Check sheet for the modelled part. Datum: model origin and axes. Units: mm. Round coordinates to 2 decimals unless told otherwise and drop trailing zeros. Order: outer loops, then holes, each group sorted by start corner. A loop starts at its lowest first (then second) coordinate and runs counter-clockwise, first axis right, second up.
```python
from build123d import *

# Parameters (mm, degrees)
F1_DEPTH     = 300
F2_R         = 15
F4_DEPTH     = 1
F5_T1_DEPTH  = 260
F5_T3_DEPTH  = 114.4173096389
F5_T5_DEPTH  = 114.4173096389
F5_T8_ANGLE  = 90
F5_T10_ANGLE = 90
F5_T12_ANGLE = 90
F5_T14_ANGLE = 90
F7_DEPTH     = 0.1
F9_DEPTH     = 0.1


# Not quite as in the source:
# - a fillet or chamfer that OpenCascade refuses, or shapes differently, is made with other operations: its cross-section is extruded or revolved along the edge and cut away or added


with BuildPart() as f1:
    # F0 (on Right) → F1 (new body)
    with BuildSketch(Plane.YZ):
        Polygon((-104.210527479, 1), (-104.210527479, 0), (115.789472521, 0), (115.789472521, 10), align=None)
    extrude(amount=F1_DEPTH)

    # F2
    f2_edges = [f1.edges().sort_by_distance(p)[0] for p in [
        (300, 115.789473, 5),
        (0, 115.789473, 5),
        (0, -104.210527, 0.5),
        (300, -104.210527, 0.5),
    ]]
    fillet(f2_edges, radius=F2_R)

    # F3 (on face) → F4 (cut)
    with BuildSketch(Plane(origin=(0, -0.2149512742, 5.2543644811), x_dir=(1, 0, 0), z_dir=(0, -0.040874902, 0.999164272))):
        with BuildLine():
            Line((280, 101.0889066279), (20, 101.0889066279))
            ThreePointArc((20, 101.0889066279), (16.4644660941, 99.6244405339), (15, 96.0889066279))
            Line((15, 96.0889066279), (15, -18.328403011))
            ThreePointArc((15, -18.328403011), (16.4644660941, -21.8639369169), (20, -23.328403011))
            Line((20, -23.328403011), (280, -23.328403011))
            ThreePointArc((280, -23.328403011), (283.5355339059, -21.8639369169), (285, -18.328403011))
            Line((285, -18.328403011), (285, 96.0889066279))
            ThreePointArc((285, 96.0889066279), (283.5355339059, 99.6244405339), (280, 101.0889066279))
        make_face()
    extrude(amount=-F4_DEPTH, mode=Mode.SUBTRACT)

    # F5: fillet of radius 5 on 8 edges, made by hand

    # F5_s2 → F5_t1 (join)
    with BuildSketch(Plane.YZ.offset(20)):
        with BuildLine():
            ThreePointArc((100.789472521, 9.3863636364), (99.4021842094, 8.5855726288), (97.8328546072, 8.2645746583))
            Line((97.8328546072, 8.2645746583), (100.8303474231, 8.3871993644))
            Line((100.8303474231, 8.3871993644), (100.789472521, 9.3863636364))
        make_face()
        with BuildLine():
            ThreePointArc((-23.5238580849, 4.3008182934), (-22.0757956208, 3.6160189085), (-20.485490367, 3.4242787275))
            Line((-20.485490367, 3.4242787275), (-23.4829831829, 3.3016540214))
            Line((-23.4829831829, 3.3016540214), (-23.5238580849, 4.3008182934))
        make_face()
    extrude(amount=F5_T1_DEPTH)

    # F5_s4 → F5_t3 (join)
    with BuildSketch(Plane(origin=(0, 96.0086024354, 3.9276246451), x_dir=(1, 0, 0), z_dir=(0, -0.999164272, -0.040874902))):
        with BuildLine():
            ThreePointArc((15, 5.2587593737), (16.4188611699, 4.5153428835), (18, 4.2587593737))
            Line((18, 4.2587593737), (15, 4.2587593737))
            Line((15, 4.2587593737), (15, 5.2587593737))
        make_face()
    extrude(amount=F5_T3_DEPTH)

    # F5_s6 → F5_t5 (join)
    with BuildSketch(Plane(origin=(0, -18.3130854508, -0.7491716775), x_dir=(1, 0, 0), z_dir=(0, 0.999164272, 0.040874902))):
        with BuildLine():
            ThreePointArc((285, -5.2587593737), (283.5811388301, -4.5153428835), (282, -4.2587593737))
            Line((282, -4.2587593737), (285, -4.2587593737))
            Line((285, -4.2587593737), (285, -5.2587593737))
        make_face()
    extrude(amount=F5_T5_DEPTH)

    # F5_s7 → F5_t8 (revolve)
    with BuildSketch(Plane.YZ.offset(20)):
        with BuildLine():
            ThreePointArc((100.789472521, 9.3863636364), (99.4021842094, 8.5855726288), (97.8328546072, 8.2645746583))
            Line((97.8328546072, 8.2645746583), (100.8303474231, 8.3871993644))
            Line((100.8303474231, 8.3871993644), (100.789472521, 9.3863636364))
        make_face()
    revolve(axis=Axis((20, 95.8345260632, 8.1828248542), (0, -0.040874902, 0.999164272)), revolution_arc=F5_T8_ANGLE)

    # F5_s9 → F5_t10 (revolve)
    with BuildSketch(Plane(origin=(0, -18.3130854508, -0.7491716775), x_dir=(1, 0, 0), z_dir=(0, 0.999164272, 0.040874902))):
        with BuildLine():
            ThreePointArc((15, -5.2587593737), (16.4188611699, -4.5153428835), (18, -4.2587593737))
            Line((18, -4.2587593737), (15, -4.2587593737))
            Line((15, -4.2587593737), (15, -5.2587593737))
        make_face()
    revolve(axis=Axis((20, -18.487161823, 3.5060285316), (0, -0.040874902, 0.999164272)), revolution_arc=F5_T10_ANGLE)

    # F5_s11 → F5_t12 (revolve)
    with BuildSketch(Plane.YZ.offset(280)):
        with BuildLine():
            ThreePointArc((-23.5238580849, 4.3008182934), (-22.0757956208, 3.6160189085), (-20.485490367, 3.4242787275))
            Line((-20.485490367, 3.4242787275), (-23.4829831829, 3.3016540214))
            Line((-23.4829831829, 3.3016540214), (-23.5238580849, 4.3008182934))
        make_face()
    revolve(axis=Axis((280, -18.487161823, 3.5060285316), (0, -0.040874902, 0.999164272)), revolution_arc=F5_T12_ANGLE)

    # F5_s13 → F5_t14 (revolve)
    with BuildSketch(Plane(origin=(0, 96.0086024354, 3.9276246451), x_dir=(1, 0, 0), z_dir=(0, -0.999164272, -0.040874902))):
        with BuildLine():
            ThreePointArc((285, 5.2587593737), (283.5811388301, 4.5153428835), (282, 4.2587593737))
            Line((282, 4.2587593737), (285, 4.2587593737))
            Line((285, 4.2587593737), (285, 5.2587593737))
        make_face()
    revolve(axis=Axis((280, 95.8345260632, 8.1828248542), (0, -0.040874902, 0.999164272)), revolution_arc=F5_T14_ANGLE)

    # F6 (on face) → F7 (cut)
    with BuildSketch(Plane(origin=(0, -0.2149512742, 5.2543644811), x_dir=(1, 0, 0), z_dir=(0, -0.040874902, 0.999164272))):
        with BuildLine():
            Line((182.0928883553, -37.4153330922), (117.9071116447, -37.4153330922))
            ThreePointArc((117.9071116447, -37.4153330922), (114.3715777388, -38.8797991863), (112.9071116447, -42.4153330922))
            Line((112.9071116447, -42.4153330922), (112.9071116447, -79.291882813))
            ThreePointArc((112.9071116447, -79.291882813), (114.3715777388, -82.8274167189), (117.9071116447, -84.291882813))
            Line((117.9071116447, -84.291882813), (182.0928883553, -84.291882813))
            ThreePointArc((182.0928883553, -84.291882813), (185.6284222612, -82.8274167189), (187.0928883553, -79.291882813))
            Line((187.0928883553, -79.291882813), (187.0928883553, -42.4153330922))
            ThreePointArc((187.0928883553, -42.4153330922), (185.6284222612, -38.8797991863), (182.0928883553, -37.4153330922))
        make_face()
    extrude(amount=-F7_DEPTH, mode=Mode.SUBTRACT)

    # F8 (on face) → F9 (cut)
    with BuildSketch(Plane(origin=(0, -0.1740763722, 4.2552002091), x_dir=(1, 0, 0), z_dir=(0, -0.040874902, 0.999164272))):
        with BuildLine():
            Line((28.5042302459, 96.0889066279), (21, 96.0889066279))
            ThreePointArc((21, 96.0889066279), (20.2928932188, 95.7960134091), (20, 95.0889066279))
            Line((20, 95.0889066279), (20, 90.473426342))
            ThreePointArc((20, 90.473426342), (20.2928932188, 89.7663195608), (21, 89.473426342))
            Line((21, 89.473426342), (28.5042302459, 89.473426342))
            ThreePointArc((28.5042302459, 89.473426342), (29.2113370271, 89.7663195608), (29.5042302459, 90.473426342))
            Line((29.5042302459, 90.473426342), (29.5042302459, 95.0889066279))
            ThreePointArc((29.5042302459, 95.0889066279), (29.2113370271, 95.7960134091), (28.5042302459, 96.0889066279))
        make_face()
    extrude(amount=-F9_DEPTH, mode=Mode.SUBTRACT)


solid = f1.part
```
Item 1: Sectioned sample at B-B (x = 51.5). Record the cut outline in (y, z).
Answer:
outline: (-104.21, 0) - (115.79, 0) - (115.79, 10) - (100.79, 9.39) arc R5 cw to (97.83, 8.26) - (-20.49, 3.42) arc R5 cw to (-23.52, 4.3) - (-104.21, 1) - close
Item 2: Sectioned sample at C-C (y = -28.5). Record the cut outline in (x, z).
Answer:
outline: (0, 0) - (300, 0) - (300, 4.1) - (0, 4.1) - close
Item 3: Go/stop test with flat-tipped pins: P1, Ø3, axis at x = 226.5, y = 70, coming from the +Z side; P2, Ø12, axis at x = 102, y = -60.5, coming from the +Z side. Record where each tip stops, or that it passes through.
Answer:
P1: stops at z = 7.19
P2: stops at z = 3.03
Item 4: Release check for a two-part mould opening along X. For faces 1 (the cylindrical face through (16.4, 39.46, 6.14)), 2 (the cylindrical face through (295.49, -99.93, 0.62)) record: released by +X, released by -X, zero draft, split by the parting line, or undercut.
Answer:
face 1: undercut
face 2: released by +X
Item 5: Scan lines: line 1 along Z through (x, y) = (23, 91); line 2 along Z through (x, y) = (249, -23.5); line 3 along Y through (x, z) = (179.5, 8.75). Record each from-to range of solid material in increasing order.
Answer:
line 1: z = 0 to 7.88
line 2: z = 0 to 4.28
line 3: y = 99.79 to 115.79
Item 6: Sectioned sample at A-A (x = 178). Record the cut outline in (y, z).
Answer:
outline: (-104.21, 0) - (115.79, 0) - (115.79, 10) - (100.79, 9.39) arc R5 cw to (97.83, 8.26) - (-20.49, 3.42) arc R5 cw to (-23.52, 4.3) - (-37.6, 3.73) - (-37.59, 3.63) - (-84.43, 1.71) - (-84.44, 1.81) - (-104.21, 1) - close
